Part print with two shaded views. Sizes in mm from the minimum x, y, z corner. Coordinates: 2 decimals unless noted, no trailing zeros. Loops run counter-clockwise (first coordinate to the right, second up) from the corner with the lowest first, then second, coordinate; pieces in that order, holes last. Notation, with made-up numbers: (-15, 38) - (33, 38) arc R27 ccw to (33, 73) - close; hole circle Ø6 at (-11.5, 51.25). An arc over 180 degrees is marked (long way). Answer as CSV lines item,"result".
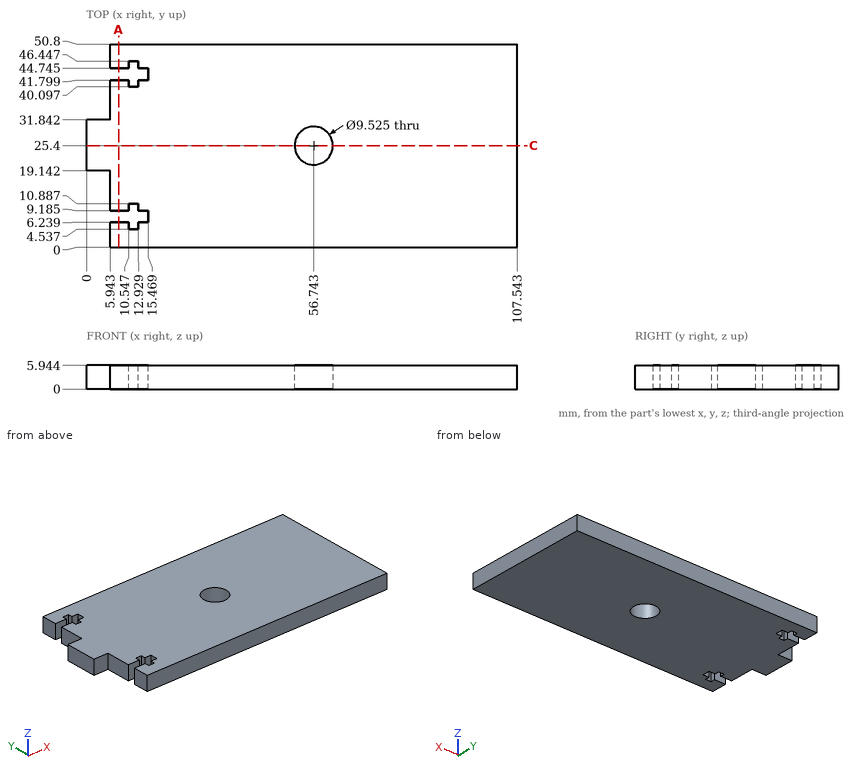
Q1. Saw through at A-A (x = 8). Give the cut face in (y, z) (1 decimal), then the cut area to 3 significant figures.
Results:
outline,"(0, 0) - (6.2, 0) - (6.2, 5.9) - (0, 5.9) - close; (9.2, 0) - (41.8, 0) - (41.8, 5.9) - (9.2, 5.9) - close; (44.7, 0) - (50.8, 0) - (50.8, 5.9) - (44.7, 5.9) - close"
area,"267 mm^2"
Q2. Saw through at C-C (y = 25.4). Give the cut face in (x, z).
Results:
outline,"(0, 0) - (51.98, 0) - (51.98, 5.94) - (0, 5.94) - close; (61.51, 0) - (107.54, 0) - (107.54, 5.94) - (61.51, 5.94) - close"
Q3. Flat gauge pin, fed straight in: pin 1 (0.9 mm diameter, centred on y = 44, z = 2.5, fed in from -X). Where does the tip first touch, or does it go through?
Results:
pin 1,"stops at x = 15.47"
Q4. Wall check: L1, parallel to Y at x = 13, z = 3.65 (1 decimal); L2, parallel to X at y = 6, z = 3.1; L3, parallel to X at y = 25.5, z = 0.35 (1 decimal). Give the ranges that are in metal, low to high.
Results:
L1,"y = 0 to 6.2, 9.2 to 41.8, 44.7 to 50.8"
L2,"x = 5.94 to 10.55, 12.93 to 107.54"
L3,"x = 0 to 52, 61.5 to 107.5"
